```python
from build123d import *

# Parameters (mm, degrees)
SCHIZZO13_R                  = 1.5
SCHIZZO13_R_2                = 2.75
ESTRUSIONE_ESTRUSIONE2_DEPTH = 5


with BuildPart() as part:
    # Schizzo13 → Estrusione-Estrusione2 (new body)
    with BuildSketch(Plane.XY):
        Polygon((10, 0), (340, 0), (350, 10), (350, 350), (0, 350), (0, 10), align=None)
        with Locations((15, 320)):
            Circle(SCHIZZO13_R, mode=Mode.SUBTRACT)
        with Locations((20.5, 279.5)):
            Circle(SCHIZZO13_R, mode=Mode.SUBTRACT)
        with Locations((70.5, 279.5)):
            Circle(SCHIZZO13_R, mode=Mode.SUBTRACT)
        with Locations((175, 175)):
            Circle(SCHIZZO13_R, mode=Mode.SUBTRACT)
        with Locations((20.5, 70.5)):
            Circle(SCHIZZO13_R, mode=Mode.SUBTRACT)
        with Locations((200, 344)):
            Circle(SCHIZZO13_R_2, mode=Mode.SUBTRACT)
        with Locations((150, 344)):
            Circle(SCHIZZO13_R_2, mode=Mode.SUBTRACT)
        with Locations((175, 329)):
            Circle(SCHIZZO13_R_2, mode=Mode.SUBTRACT)
        with Locations((217, 329)):
            Circle(SCHIZZO13_R_2, mode=Mode.SUBTRACT)
        with Locations((133, 329)):
            Circle(SCHIZZO13_R_2, mode=Mode.SUBTRACT)
        with Locations((70.5, 70.5)):
            Circle(SCHIZZO13_R, mode=Mode.SUBTRACT)
        with Locations((279.5, 70.5)):
            Circle(SCHIZZO13_R, mode=Mode.SUBTRACT)
        with Locations((329.5, 70.5)):
            Circle(SCHIZZO13_R, mode=Mode.SUBTRACT)
        with Locations((335, 10)):
            Circle(SCHIZZO13_R, mode=Mode.SUBTRACT)
        with Locations((15, 10)):
            Circle(SCHIZZO13_R, mode=Mode.SUBTRACT)
        with Locations((279.5, 279.5)):
            Circle(SCHIZZO13_R, mode=Mode.SUBTRACT)
        with Locations((329.5, 279.5)):
            Circle(SCHIZZO13_R, mode=Mode.SUBTRACT)
        with Locations((335, 320)):
            Circle(SCHIZZO13_R, mode=Mode.SUBTRACT)
        with Locations((295, 344)):
            Circle(SCHIZZO13_R, mode=Mode.SUBTRACT)
        with Locations((315, 344)):
            Circle(SCHIZZO13_R, mode=Mode.SUBTRACT)
    extrude(amount=-ESTRUSIONE_ESTRUSIONE2_DEPTH)


solid = part.part
```
Check sheet for the modelled part. Datum: model origin and axes. Units: mm. Coordinates: 2 decimals unless noted, no trailing zeros. Write item = value, one per line. Start each with the question number.
1) Mould release check, pull along X, two halves, no side actions. Record for faces 1 (the flat face through (345, 5, -2)), 2 (the flat face through (173, 177, 0)), 3 (the flat face through (5, 5, -2)): +X half, -X half, draft (parallel to the pull), parting line (faces both ways), or undercut.
2) Material ranges on L1, parallel to X at y = 329, z = -1.15; L2, parallel to X at y = 344, z = -2.45; L3, parallel to X at y = 70.5, z = -3.4, recorded low to high.
3) Go/stop test with a flat-tipped pin: P1, Ø1.8, axis at x = 20.5, y = 70.5, coming from the +Z side. Record where the tip stops, or that it passes through.
Ans:
q1.face_1 = +X half
q1.face_2 = draft
q1.face_3 = -X half
q2.L1 = 0 to 130.25, 135.75 to 172.25, 177.75 to 214.25, 219.75 to 350
q2.L2 = 0 to 147.25, 152.75 to 197.25, 202.75 to 293.5, 296.5 to 313.5, 316.5 to 350
q2.L3 = 0 to 19, 22 to 69, 72 to 278, 281 to 328, 331 to 350
q3.P1 = through
